from build123d import *

# Parameters (mm, degrees)
PAD_DEPTH       = 2
SKETCH001_W     = 88
SKETCH001_H     = 20.999999
POCKET_DEPTH    = 5
SKETCH002_R     = 1.45
POCKET001_DEPTH = 5
SKETCH005_R     = 1.45
PAD001_DEPTH    = 20
FILLET_R        = 1.5


with BuildPart() as part:
    # Sketch → Pad (new body)
    with BuildSketch(Plane.XY):
        with BuildLine():
            Line((-50.000004, 29.999999), (49.999993, 29.999999))
            ThreePointArc((49.999993, -29.999999), (71.628774, 0), (49.999993, 29.999999))
            Line((-50.000004, -29.999999), (49.999993, -29.999999))
            ThreePointArc((-50.000004, 29.999999), (-71.628785, 0), (-50.000004, -29.999999))
        make_face()
    extrude(amount=PAD_DEPTH)

    # Sketch001 (on Face6 of Pad) → Pocket (cut)
    with BuildSketch(Plane.XY.offset(2)):
        with Locations((6, 19.5)):
            Rectangle(SKETCH001_W, SKETCH001_H)
    extrude(amount=-POCKET_DEPTH, mode=Mode.SUBTRACT)

    # Sketch002 (on Face5 of Pocket) → Pocket001 (cut)
    with BuildSketch(Plane.XY.offset(2)):
        with Locations((-56, 22)):
            Circle(SKETCH002_R)
        with Locations((-56, -22)):
            Circle(SKETCH002_R)
        with Locations((56, 22)):
            Circle(SKETCH002_R)
        with Locations((56, -22)):
            Circle(SKETCH002_R)
    extrude(amount=-POCKET001_DEPTH, mode=Mode.SUBTRACT)

    # Sketch005 (on Sketch) → Pad001 (join)
    with BuildSketch(Plane(origin=(0, 0, 0), x_dir=(1, 0, 0), z_dir=(0, 0, -1))):
        with BuildLine():
            ThreePointArc((57.824475, -21.180678), (66.188679, -0.02241), (57.855075, 21.147928))
            ThreePointArc((57.855075, 21.147928), (57.421669, 23.451415), (55.098354, 23.761422))
            ThreePointArc((55.098354, 23.761422), (49.395322, 27.553068), (42.998941, 29.999999))
            Line((42.998941, 29.999999), (-42.810254, 29.999999))
            ThreePointArc((-42.810254, 29.999999), (-49.250438, 27.530438), (-54.985149, 23.697971))
            ThreePointArc((-54.985149, 23.697971), (-57.424375, 23.445333), (-57.785293, 21.019763))
            ThreePointArc((-57.785293, 21.019763), (-65.999994, -0.019369), (-57.759009, -21.048219))
            ThreePointArc((-57.759009, -21.048219), (-54.555317, -23.383073), (-57.02749, -20.284114))
            ThreePointArc((-57.042198, 20.268075), (-64.924214, -0.010881), (-57.02749, -20.284114))
            ThreePointArc((-57.042198, 20.268075), (-54.656994, 20.557152), (-54.270591, 22.928536))
            ThreePointArc((-42.606362, 28.999735), (-48.775213, 26.611086), (-54.270591, 22.928536))
            Line((-42.606362, 28.999735), (42.682146, 28.999735))
            ThreePointArc((54.296791, 22.970282), (48.822241, 26.626033), (42.682146, 28.999735))
            ThreePointArc((54.296791, 22.970282), (54.663143, 20.554788), (57.0925, 20.295848))
            ThreePointArc((57.075816, -20.313993), (64.999997, -0.012324), (57.0925, 20.295848))
            ThreePointArc((57.075816, -20.313993), (54.486491, -23.307399), (57.824475, -21.180678))
        make_face()
        with Locations((-56.041981, 22)):
            Circle(SKETCH005_R, mode=Mode.SUBTRACT)
        with Locations((56.045663, 22)):
            Circle(SKETCH005_R, mode=Mode.SUBTRACT)
        with Locations((56, -22)):
            Circle(SKETCH005_R, mode=Mode.SUBTRACT)
        with Locations((-56, -22)):
            Circle(SKETCH005_R, mode=Mode.SUBTRACT)
    extrude(amount=PAD001_DEPTH)

    # Fillet
    fillet_edges = [part.edges().sort_by_distance(p)[0] for p in [
        (-71.628785, 0, 2),
        (-44.000002, 29.999999, 2),
        (-5e-06, -29.999999, 2),
        (71.628774, -4e-06, 2),
    ]]
    fillet(fillet_edges, radius=FILLET_R)


solid = part.part
Check sheet for the modelled part. Datum: model origin and axes. Units: mm. A direction names the side the tool comes from. Give positions to 0.01 mm unless a question says otherwise; leave off trailing zeros. Write each loop counter-clockwise with the first axis right and the second up, starting at its lowest first coordinate (ties: lowest second). Pieces come first, ordered by that corner, then holes. Notation, with made-up numbers: (-29.75, 60.25) -> (5.25, 60.25) arc R22 ccw to (5.25, 71.25) -> close; hole circle Ø10 at (39, -14.75). An arc over 180 degrees is marked (long way). Use one line per item in the form item = value. Start each with the question number.
1. Access from +Z, -Z, +X, -X, +Y, -Y to the whole of each face (thin tool, end or side, straight path). Record for faces 4 (the flat face through (1, -6, 2)), 5 (the cylindrical face through (66.187, 0.349, -9.86)), 6 (the cylindrical face through (-57.4, -23.47, -9.86)).
2. Section check C-C (x = -45.5). Record the cut outline in (y, z), and give its area (3 significant figures).
3. Mould release check, pull along Y, two halves, no side actions. Record for faces 1 (the cylindrical face through (-57.45, 21.94, -8.85)), 2 (the cylindrical face through (71.624, -0.553, 0.247)), 3 (the flat face through (-1, -29, -10)): pulls with the +Y half, pulls with the -Y half, needs draft (parallel to the pull), parting line crosses it, or undercut.
4. Thickness scan on line 1 along Y through (x, z) = (-56, -3.5); line 2 along X through (y, z) = (-22, -11); line 3 along X through (y, z) = (22, -2.25). Record the ranges inside material, lowest first. Write a range as from..to.
5. Go/stop test with flat-tipped pins: P1, Ø1.6, axis at x = 5, z = 1.5, coming from the +Y side; P2, Ø2, axis at x = 17, z = -7.5, coming from the +Y side; P3, Ø0.7, axis at x = 56.5, y = -22.5, coming from the -Z side; P4, Ø5, axis at y = 17.5, z = -14, coming from the -X side. Record where each tip stops, or that it passes through.
6. Section check B-B (z = -15.5). Record the cut outline in (x, y).
7. Section check A-A (x = -5). Record the cut outline in (y, z), and give its area (3 significant figures).
Conclusion:
q1.face_4 = +Z, +X, -X, +Y, -Y
q1.face_5 = -Z, +X
q1.face_6 = -Z
q2.outline = (-30, 0) -> (-29.17, 0) -> (-29.17, -20) -> (-28.07, -20) -> (-28.07, 0) -> (30, 0) -> (30, 0.5) arc R1.5 ccw to (28.5, 2) -> (-28.5, 2) arc R1.5 ccw to (-30, 0.5) -> close
q2.area = 141 mm²
q3.face_1 = undercut
q3.face_2 = parting line crosses it
q3.face_3 = pulls with the +Y half
q4.line_1 = -24..-23.45, -20.55..-20, 20..20.55, 23.45..24
q4.line_2 = -58.04..-57.49, -54.59..-54.04, 54.05..54.6, 57.5..58.05
q4.line_3 = -58..-57.45, -54.55..-54, 54..54.55, 57.45..58
q5.P1 = 9
q5.P2 = -29
q5.P3 = through
q5.P4 = -62.13
q6.outline = (-57.79, -21.02) arc R2 ccw to (-54.99, -23.7) arc R31 ccw to (-42.81, -30) -> (43, -30) arc R31 ccw to (55.1, -23.76) arc R2 ccw to (57.86, -21.15) arc R31 ccw to (57.82, 21.18) arc R2 ccw (long way) to (57.08, 20.31) arc R30 cw to (57.09, -20.3) arc R2 ccw to (54.3, -22.97) arc R30 cw to (42.68, -29) -> (-42.61, -29) arc R30 cw to (-54.27, -22.93) arc R2 ccw to (-57.04, -20.27) arc R30 cw to (-57.03, 20.28) arc R2 ccw (long way) to (-57.76, 21.05) arc R31 ccw to start; hole circle Ø2.9 at (-56.04, -22); hole circle Ø2.9 at (-56, 22); hole circle Ø2.9 at (56, 22); hole circle Ø2.9 at (56.05, -22)
q7.outline = (-30, -20) -> (-29, -20) -> (-29, 0) -> (9, 0) -> (9, 2) -> (-28.5, 2) arc R1.5 ccw to (-30, 0.5) -> close
q7.area = 97.5 mm²
